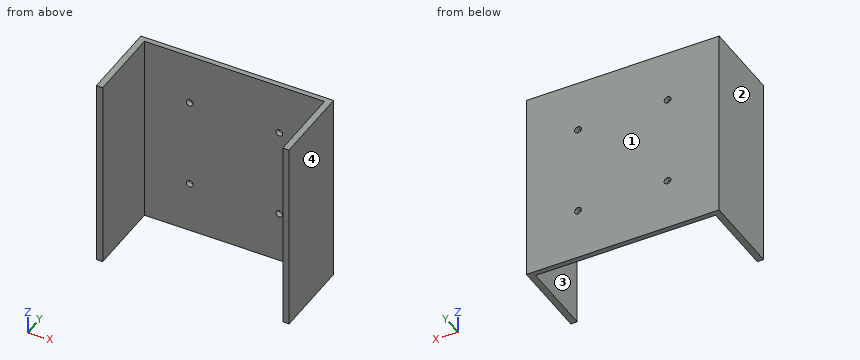
```python
from build123d import *

# Parameters (mm, degrees)
SKETCH1_W           = 96.52
SKETCH1_H           = 96.52
SKETCH1_R           = 1.7
BOSS_EXTRUDE1_DEPTH = 2.54
SKETCH2_W           = 3.175
SKETCH2_H           = 96.52
BOSS_EXTRUDE2_DEPTH = 38.1


with BuildPart() as part:
    # Sketch1 → Boss-Extrude1 (new body)
    with BuildSketch(Plane(origin=(0, 0, 0), x_dir=(1, 0, 0), z_dir=(0, 1, 0))):
        Rectangle(SKETCH1_W, SKETCH1_H)
        with Locations((-22.447883068, 22.447883068)):
            Circle(SKETCH1_R, mode=Mode.SUBTRACT)
        with Locations((22.447883068, 22.447883068)):
            Circle(SKETCH1_R, mode=Mode.SUBTRACT)
        with Locations((22.447883068, -22.447883068)):
            Circle(SKETCH1_R, mode=Mode.SUBTRACT)
        with Locations((-22.447883068, -22.447883068)):
            Circle(SKETCH1_R, mode=Mode.SUBTRACT)
    extrude(amount=BOSS_EXTRUDE1_DEPTH)

    # Sketch2 → Boss-Extrude2 (add)
    with BuildSketch(Plane.XZ):
        with Locations((-46.6725, 0)):
            Rectangle(SKETCH2_W, SKETCH2_H)
        with Locations((46.6725, 0)):
            Rectangle(SKETCH2_W, SKETCH2_H)
    extrude(amount=BOSS_EXTRUDE2_DEPTH)


solid = part.part
```
Here's how the part is built. I have some questions about the finished solid (model axes, mm). Face numbers are marked on the shaded views. Give positions to 0.01 mm unless a question says otherwise; leave off trailing zeros. Order: outer loops, then holes, each group sorted by start corner. A loop starts at its lowest first (then second) coordinate and runs counter-clockwise, first axis right, second up. Notation, with made-up numbers: M 28.25,36 L 32.25,36 A31 ccw 32.25,61 Z; hole C -39.75,31 d8. An arc over 180 degrees is marked long. Use a Markdown table: item, result. Add a question column.
1. Suppose I cut it at C-C (x = 26.5). List the corners of the cut face in (y, z) for me.
2. Suppose I cut it at A-A (y = -28.5). List the corners of the cut face in (x, z) for me (3 decimals).
3. If we mould it in two halves opening along X, with no side actions, what happens to the marked faces 1, 2, 3 and 4? For each: +X half, -X half, draft (parallel to the pull), parting line (faces both ways), or undercut.
4. For pin 1 Ø4.5 at (x, z) = (22.45, -22.45) entering from -Y, with a flat end and sliding along its axis, tell me the tip position at first contact or that it passes through.
5. Suppose I cut it at B-B (z = 18). List the corners of the cut face in (x, y) for me (3 decimals), and give its area (3 significant figures).
6. I need wall thicknesses on probe 1 along X at (y, z) = (-12, 2) (3 decimals); probe 2 along Z at (x, y) = (-21.5, 0.5); probe 3 along Y at (x, z) = (-21, -29). Which ranges of each line are inside material? Lowest first, please. Write a range as from..to.
Results list:
| question | item | result |
|---|---|---|
| 1 | outline | M 0,-48.26 L 2.54,-48.26 L 2.54,48.26 L 0,48.26 Z |
| 2 | outline | M -48.26,-48.26 L -45.085,-48.26 L -45.085,48.26 L -48.26,48.26 Z; M 45.085,-48.26 L 48.26,-48.26 L 48.26,48.26 L 45.085,48.26 Z |
| 3 | face 1 | draft |
| 3 | face 2 | -X half |
| 3 | face 3 | undercut |
| 3 | face 4 | +X half |
| 4 | pin 1 | stops at y = 0 |
| 5 | outline | M -48.26,-38.1 L -45.085,-38.1 L -45.085,0 L 45.085,0 L 45.085,-38.1 L 48.26,-38.1 L 48.26,2.54 L -48.26,2.54 Z |
| 5 | area | 487 mm² |
| 6 | probe 1 | x = -48.26..-45.085, 45.085..48.26 |
| 6 | probe 2 | z = -48.26..-23.86, -21.04..21.04, 23.86..48.26 |
| 6 | probe 3 | y = 0..2.54 |
